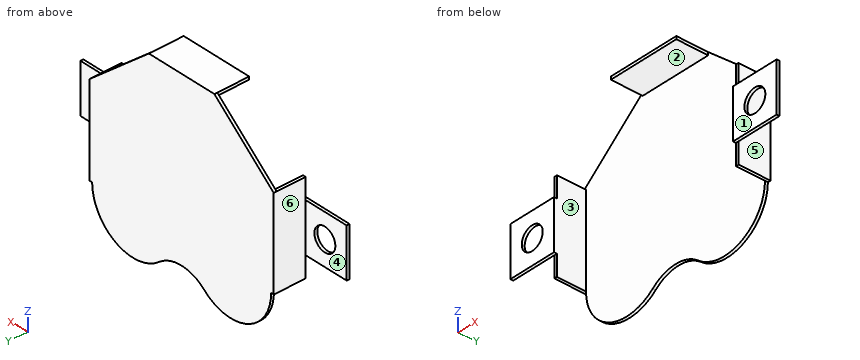
```python
from build123d import *

# Parameters (mm, degrees)
SKETCH1_W             = 5
SKETCH1_H             = 5.1
SKETCH1_R             = 1.2
BOSS_EXTRUDE1_DEPTH   = 0.3
BOSS_EXTRUDE1_2_DEPTH = 0.3
SKETCH1_W_2           = 7.5
SKETCH1_H_2           = 0.3
BOSS_EXTRUDE1_3_DEPTH = 0.3
SKETCH2_W             = 0.3
SKETCH2_H             = 9.4
SKETCH2_W_2           = 7.5
SKETCH2_H_2           = 0.3
BOSS_EXTRUDE2_DEPTH   = 3
BOSS_EXTRUDE3_DEPTH   = 0.3


with BuildPart() as part:
    # Sketch1 → Boss-Extrude1 (new body)
    with BuildSketch(Plane(origin=(0, 0, 0), x_dir=(1, 0, 0), z_dir=(0, 1, 0))):
        with Locations((-12.75, 0)):
            Rectangle(SKETCH1_W, SKETCH1_H)
        with Locations(Location((-12.75, 0, 0), (0, 0, 270))):
            Circle(SKETCH1_R, mode=Mode.SUBTRACT)
    extrude(amount=BOSS_EXTRUDE1_DEPTH)



with BuildPart() as body_2:
    # Sketch1 → Boss-Extrude1 2 (new body)
    with BuildSketch(Plane(origin=(0, 0, 0), x_dir=(1, 0, 0), z_dir=(0, 1, 0))):
        with Locations((12.75, 0)):
            Rectangle(SKETCH1_W, SKETCH1_H)
        with Locations(Location((12.75, 0, 0), (0, 0, 270))):
            Circle(SKETCH1_R, mode=Mode.SUBTRACT)
    extrude(amount=BOSS_EXTRUDE1_2_DEPTH)


with BuildPart() as body_3:
    # Sketch1 → Boss-Extrude1 3 (new body)
    with BuildSketch(Plane(origin=(0, 0, 0), x_dir=(1, 0, 0), z_dir=(0, 1, 0))):
        with Locations((0, -10.3)):
            Rectangle(SKETCH1_W_2, SKETCH1_H_2)
    extrude(amount=BOSS_EXTRUDE1_3_DEPTH)


with BuildPart() as part_1:
    add(part.part)

    add(body_2.part)  # Boss-Extrude2 merges body 2

    add(body_3.part)  # Boss-Extrude2 merges body 3
    # Sketch2 → Boss-Extrude2 (add)
    with BuildSketch(Plane(origin=(0, 0.3, 0), x_dir=(1, 0, 0), z_dir=(0, 1, 0))):
        with Locations((-10.4, 0)):
            Rectangle(SKETCH2_W, SKETCH2_H)
        with Locations((10.4, 0)):
            Rectangle(SKETCH2_W, SKETCH2_H)
        with Locations((0, -10.3)):
            Rectangle(SKETCH2_W_2, SKETCH2_H_2)
    extrude(amount=BOSS_EXTRUDE2_DEPTH)

    # Sketch3 → Boss-Extrude3 (add)
    with BuildSketch(Plane(origin=(0, 3.3, 0), x_dir=(1, 0, 0), z_dir=(0, 1, 0))):
        with BuildLine():
            Line((-3.75, -10.45), (-10.55, -4.7))
            Line((-10.55, -4.7), (-10.55, 4.7))
            Line((-10.55, 4.7), (-10.25, 4.7))
            ThreePointArc((-10.25, 4.7), (-7.551234557, 8.92080368), (-2.587555397, 8.242270108))
            ThreePointArc((-2.587555397, 8.242270108), (0, 7.290779594), (2.587555397, 8.242270108))
            ThreePointArc((2.587555397, 8.242270108), (7.551234557, 8.92080368), (10.25, 4.7))
            Line((10.25, 4.7), (10.55, 4.7))
            Line((10.55, 4.7), (10.55, -4.7))
            Line((10.55, -4.7), (3.75, -10.45))
            Line((3.75, -10.45), (-3.75, -10.45))
        make_face()
    extrude(amount=BOSS_EXTRUDE3_DEPTH)


solid = part_1.part
```
Work out the finished part from the listing and answer in its coordinate system (mm). Face numbers are marked on the shaded views. A direction names the side the tool comes from. Give positions to 0.01 mm unless a question says otherwise; leave off trailing zeros. Loops run counter-clockwise (first coordinate to the right, second up) from the corner with the lowest first, then second, coordinate; pieces in that order, holes last. Notation, with made-up numbers: M 17.5,25.5 L 64.5,25.5 A16 ccw 64.5,49.5 Z; hole C -2,57.5 d1. An arc over 180 degrees is marked long. One line per item, written item: value. Start each with the question number.
1. Find section B-B (z = 0). Give the vertices of the cut face in (x, y).
2. Each of these flat-tipped pins is pushed along its axis until it touches: P1, Ø2, axis at x = -11.5, y = 1.5, coming from the -Z side; P2, Ø6, axis at x = -7, z = -3, coming from the -Y side; P3, Ø1.4, axis at x = 13.5, z = 0.5, coming from the +Y side. Where does it stop, or does it pass through?
3. Which of the six approach directions +Z, -Z, +X, -X, +Y, -Y give full straight-line access (tool end or side, diameter ignored) to the marked faces 1 and 2?
4. Find section A-A (y = 1.25). Give the vertices of the cut face in (x, z).
5. Find section D-D (z = -4.25). Give the vertices of the cut face in (x, y).
6. Find section C-C (x = 12.75). Give the vertices of the cut face in (y, z), and give its area (3 significant figures).
7. Find the intervals of material crossed by probe 1 along X at (y, z) = (0.25, 0); probe 2 along Y at (x, z) = (1.5, -5.75); probe 3 along Z at (x, y) = (2, 1.5), in increasing order.
8. Determine the mould class of the marked faces 3, 4, 5 and 6 for opening direction X: released by +X, released by -X, zero draft, split by the parting line, or undercut.
Reported:
1. outline: M -15.25,0 L -13.95,0 L -13.95,0.3 L -15.25,0.3 Z; M -11.55,0 L -10.25,0 L -10.25,3.3 L 10.25,3.3 L 10.25,0 L 11.55,0 L 11.55,0.3 L 10.55,0.3 L 10.55,3.6 L -10.55,3.6 L -10.55,0.3 L -11.55,0.3 Z; M 13.95,0 L 15.25,0 L 15.25,0.3 L 13.95,0.3 Z
2. P1: stops at z = -4.7
2. P2: stops at y = 3.3
2. P3: stops at y = 0.3
3. face 1: +Z, -Z, +X, -X, -Y
3. face 2: -Z, +X, -X, -Y
4. outline: M -10.55,-4.7 L -10.25,-4.7 L -10.25,4.7 L -10.55,4.7 Z; M -3.75,10.15 L 3.75,10.15 L 3.75,10.45 L -3.75,10.45 Z; M 10.25,-4.7 L 10.55,-4.7 L 10.55,4.7 L 10.25,4.7 Z
5. outline: M -10.55,0.3 L -10.25,0.3 L -10.25,3.3 L 10.25,3.3 L 10.25,0.3 L 10.55,0.3 L 10.55,3.6 L -10.55,3.6 Z
6. outline: M 0,-2.55 L 0.3,-2.55 L 0.3,-1.2 L 0,-1.2 Z; M 0,1.2 L 0.3,1.2 L 0.3,2.55 L 0,2.55 Z
6. area: 0.810 mm²
7. probe 1: x = -15.25 to -13.95, -11.55 to -10.25, 10.25 to 11.55, 13.95 to 15.25
7. probe 2: y = 3.3 to 3.6
7. probe 3: z = 10.15 to 10.45
8. face 3: undercut
8. face 4: zero draft
8. face 5: released by +X
8. face 6: released by -X
